For this review, take the finished solid that the model builds, in its own axes (mm). A direction names the side the tool comes from. Coordinates: 2 decimals unless noted, no trailing zeros. Write each loop counter-clockwise with the first axis right and the second up, starting at its lowest first coordinate (ties: lowest second). Pieces come first, ordered by that corner, then holes.
1) We need section B-B on x = -35. Write out the cut boundary in (y, z) (1 decimal).
2) Insertion check: P1, Ø12, axis at y = 22, z = 12, coming from the +X side; P2, Ø6.5, axis at x = 44.5, z = 4.8, coming from the +Y side; P3, Ø0.6, axis at x = 43.5, z = 9.5, coming from the -Y side. Each pin has a flat end and moves straight along its axis. Give the tip position at first contact, or say it passes through.
3) We need section C-C on x = 44.5. Write out the cut boundary in (y, z).
4) We need section D-D on x = -7.5. Write out the cut boundary in (y, z).
5) Mouldability with a two-part tool opening along Z and no side actions: class faces 4 (the face through (-12, 0, 10)), 5 (the face through (-25.97, 21.06, 12.21)), 6 (the face through (19, 2, -2.4)) as pulls with the +Z half, pulls with the -Z half, needs draft (parallel to the pull), parting line crosses it, or undercut.
6) For faces 1 (the face through (-34, 14, 1.6)), 2 (the face through (-9, 1, 10)), 3 (the face through (-41, 22, 9)), list the 3-axis set-ups (+Z, -Z, +X, -X, +Y, -Y) from which the entire face can be reached by the end or side of a thin tool; tool diameter is ignored.
7) We need section A-A on x = 25.5. Write out the cut boundary in (y, z), then the cut area to 3 significant figures.
8) To check wall thickness, follow line 1 along X through (y, z) = (6.5, 10); line 2 along X through (y, z) = (27.25, 10); line 3 along Z through (x, y) = (-40, 3.5). State the ranges of each line that lie inside material, in increasing order.
from build123d import *

# Parameters (mm, degrees)
SKETCH1_R           = 2
BOSS_EXTRUDE1_DEPTH = 5
SKETCH2_W           = 2
SKETCH2_H           = 4
CUT_EXTRUDE1_DEPTH  = 63.375956906
BOSS_EXTRUDE2_DEPTH = 28.625
FILLET1_R           = 10
CUT_EXTRUDE2_DEPTH  = 36.25
CUT_EXTRUDE3_REACH  = 73.653
SKETCH5_R           = 5
FILLET4_R           = 10
SKETCH8_R           = 3
CUT_EXTRUDE6_DEPTH  = 22
SKETCH9_R           = 1.25
CUT_EXTRUDE7_DEPTH  = 59.195876265
FILLET5_R           = 2


with BuildPart() as part:
    # Sketch1 → Boss-Extrude1 (new body)
    with BuildSketch(Plane(origin=(0, 0, 0), x_dir=(1, 0, 0), z_dir=(0, 1, 0))):
        Polygon((-9, 2.4), (-9, 0), (-9, -22.4), (49, -22.4), (49, 2.4), align=None)
        with Locations(Location((-4.5, -15.2, 0), (0, 0, 270))):
            Circle(SKETCH1_R, mode=Mode.SUBTRACT)
        with Locations(Location((44.5, -15.2, 0), (0, 0, 270))):
            Circle(SKETCH1_R, mode=Mode.SUBTRACT)
        with Locations(Location((-4.5, -4.8, 0), (0, 0, 270))):
            Circle(SKETCH1_R, mode=Mode.SUBTRACT)
        Polygon((0, -4.8), (0, 0), (20, 0), (40, 0), (40, -10), (40, -20), (20, -20), (0, -20), (0, -10), align=None, mode=Mode.SUBTRACT)
        with Locations(Location((44.5, -4.8, 0), (0, 0, 270))):
            Circle(SKETCH1_R, mode=Mode.SUBTRACT)
    extrude(amount=BOSS_EXTRUDE1_DEPTH)

    # Sketch2 → Cut-Extrude1 (cut, through all)
    with BuildSketch(Plane.ZY.offset(9)):
        with Locations((10, 0)):
            Rectangle(SKETCH2_W, SKETCH2_H)
    extrude(amount=-CUT_EXTRUDE1_DEPTH, mode=Mode.SUBTRACT)

    # Sketch3 → Boss-Extrude2 (add)
    with BuildSketch(Plane.XZ):
        Polygon((-9, 1.6), (-9, 10), (-9, 11), (-9, 18.4), (-49, 18.4), (-49, 1.6), align=None)
    extrude(amount=-BOSS_EXTRUDE2_DEPTH)

    # Fillet1
    # the kernel refuses this fillet: 10 mm, written as the material it takes off along each edge
    with BuildSketch(Plane(origin=(-9, -20, 22.4), x_dir=(0, 0, -1), z_dir=(0, 1, 0))) as fillet1_piece_1:
        with BuildLine():
            CenterArc((10, -8), FILLET1_R, 126.869897646, 53.130102354)
            Line((0, -8), (-0.2, -8))
            Line((-0.2, -8), (-0.2, 0))
            Line((-0.2, 0), (0, 0.2))
            ThreePointArc((0, 0.2), (2, 0.2), (3.88, 0.16))
            Line((3.88, 0.16), (4, 0))
        make_face()
    extrude(amount=45, mode=Mode.SUBTRACT)
    with BuildSketch(Plane(origin=(-9, -20, -2.4), x_dir=(0, 0, 1), z_dir=(0, 1, 0))) as fillet1_piece_2:
        with BuildLine():
            CenterArc((10, 8), FILLET1_R, 180, 53.130102354)
            Line((0, 8), (-0.2, 8))
            Line((-0.2, 8), (-0.2, 0))
            Line((-0.2, 0), (0, -0.2))
            ThreePointArc((0, -0.2), (2, -0.2), (3.88, -0.16))
            Line((3.88, -0.16), (4, 0))
        make_face()
    extrude(amount=45, mode=Mode.SUBTRACT)
    with BuildSketch(Plane(origin=(49, -25, -2.4), x_dir=(-1, 0, 0), z_dir=(0, 1, 0)), Plane(origin=(49, -25, 22.4), x_dir=(0, 0, -1), z_dir=(0, 1, 0))) as fillet1_piece_3:
        with BuildLine():
            CenterArc((FILLET1_R, FILLET1_R), FILLET1_R, 180, 90)
            Line((0, FILLET1_R), (-FILLET1_R * 0.02, FILLET1_R))
            Line((-FILLET1_R * 0.02, FILLET1_R), (-FILLET1_R * 0.02, -FILLET1_R * 0.02))
            Line((-FILLET1_R * 0.02, -FILLET1_R * 0.02), (FILLET1_R, -FILLET1_R * 0.02))
            Line((FILLET1_R, -FILLET1_R * 0.02), (FILLET1_R, 0))
        make_face()
    extrude(amount=55, mode=Mode.SUBTRACT)

    # Sketch4 → Cut-Extrude2 (cut)
    with BuildSketch(Plane.ZY.offset(49)):
        with BuildLine():
            ThreePointArc((16.1, 14.3125), (13.031141398, 19.606098193), (6.912399402, 19.573367091))
            Line((6.912399402, 19.573367091), (13.087600598, 9.051632909))
            ThreePointArc((13.087600598, 9.051632909), (15.293598193, 11.281358602), (16.1, 14.3125))
        make_face()
        with BuildLine():
            Line((13.087600598, 9.051632909), (6.912399402, 19.573367091))
            ThreePointArc((6.912399402, 19.573367091), (4.739132909, 11.224899402), (13.087600598, 9.051632909))
        make_face()
    extrude(amount=-CUT_EXTRUDE2_DEPTH, mode=Mode.SUBTRACT)

    # Sketch5 → Cut-Extrude3 (cut, up to next)
    with BuildSketch(Plane.ZY.offset(12.75), mode=Mode.PRIVATE) as cut_extrude3_sk1:
        with Locations((10, 14.3125)):
            Circle(SKETCH5_R)
    cut_extrude3_tool1 = extrude(cut_extrude3_sk1.sketch, amount=-CUT_EXTRUDE3_REACH, mode=Mode.PRIVATE) & part.part
    add(cut_extrude3_tool1.solids().sort_by_distance((-12.75, 14.3125, 10))[0], mode=Mode.SUBTRACT)

    # Fillet4
    # the kernel refuses this fillet: 10 mm, written as the material it takes off along each edge
    with BuildSketch(Plane(origin=(-9, 53.625, 1.6), x_dir=(-1, 0, 0), z_dir=(0, -1, 0))) as fillet4_piece_1:
        with BuildLine():
            CenterArc((FILLET4_R, -FILLET4_R), FILLET4_R, 90, 90)
            Line((0, -FILLET4_R), (0, 0))
            Line((0, 0), (FILLET4_R, 0))
        make_face()
    extrude(amount=48.625, mode=Mode.SUBTRACT)
    with BuildSketch(Plane(origin=(-9, 5, 18.4), x_dir=(0, 0, -1), z_dir=(0, 1, 0))) as fillet4_piece_2:
        with BuildLine():
            CenterArc((FILLET4_R, FILLET4_R), FILLET4_R, 180, 90)
            Line((0, FILLET4_R), (0, 0))
            Line((0, 0), (FILLET4_R, 0))
        make_face()
    extrude(amount=48.625, mode=Mode.SUBTRACT)

    # Sketch8 → Cut-Extrude6 (cut)
    with BuildSketch(Plane.XZ):
        with Locations(Location((-40, 10, 0), (0, 0, 270))):
            Circle(SKETCH8_R)
        with Locations(Location((-28, 10, 0), (0, 0, 270))):
            Circle(SKETCH8_R)
        with Locations(Location((-16, 10, 0), (0, 0, 270))):
            Circle(SKETCH8_R)
    extrude(amount=-CUT_EXTRUDE6_DEPTH, mode=Mode.SUBTRACT)

    # Sketch9 → Cut-Extrude7 (cut, through all)
    with BuildSketch(Plane.XZ.offset(-22)):
        with Locations(Location((-40, 10, 0), (0, 0, 270))):
            Circle(SKETCH9_R)
        with Locations(Location((-28, 10, 0), (0, 0, 270))):
            Circle(SKETCH9_R)
        with Locations(Location((-16, 10, 0), (0, 0, 270))):
            Circle(SKETCH9_R)
    extrude(amount=-CUT_EXTRUDE7_DEPTH, mode=Mode.SUBTRACT)

    # Fillet5
    fillet5_edges = [part.edges().sort_by_distance(p)[0] for p in [
        (-49, 9.051632909, 13.087600598),
    ]]
    fillet(fillet5_edges, radius=FILLET5_R)


solid = part.part
Result:
1. outline: (0, 1.6) - (28.6, 1.6) - (28.6, 18.4) - (0, 18.4) - close; hole circle Ø12.2 at (14.3, 10)
2. P1: stops at x = -9.13
2. P2: stops at y = 5
2. P3: stops at y = 2
3. outline: (0, -0.75) - (5, -0.75) - (5, 2.8) - (0, 2.8) - close; (0, 6.8) - (5, 6.8) - (5, 13.2) - (0, 13.2) - (0, 11) - (2, 11) - (2, 9) - (0, 9) - close; (0, 17.2) - (5, 17.2) - (5, 20.75) - (0, 20.75) - close
4. outline: (0, 0) - (5, 0) - (5, 20) - (0, 20) - (0, 11) - (2, 11) - (2, 9) - (0, 9) - close
5. face 4: needs draft
5. face 5: undercut
5. face 6: pulls with the -Z half
6. face 1: -Z, -X, +Y, -Y
6. face 2: +X, -Y
6. face 3: -Y
7. outline: (0, -2.4) - (5, -2.4) - (5, 0) - (0, 0) - close; (0, 20) - (5, 20) - (5, 22.4) - (0, 22.4) - close
7. area: 24.0 mm2
8. line 1: x = -48.98 to -43, -37 to -31, -25 to -19, -13 to -9.13
8. line 2: x = -49 to -41.25, -38.75 to -29.25, -26.75 to -17.25, -14.75 to -9.13
8. line 3: z = 1.6 to 7, 13 to 18.4
